```python
from build123d import *

# Parameters (mm, degrees)
SKETCH_1_W          = 20
SKETCH_1_H          = 30
SKETCH_1_W_2        = 18
SKETCH_1_H_2        = 28
EXTRUDE_1_DEPTH     = 105
CUT_EXTRUDE_1_REACH = 111.659
SKETCH_2_R          = 1.5
CUT_EXTRUDE_3_REACH = 109.935
SKETCH_5_R          = 11


with BuildPart() as part:
    # 草图1 → 拉伸-薄壁1 (new body)
    with BuildSketch(Plane.XY):
        Rectangle(SKETCH_1_W, SKETCH_1_H)
        Rectangle(SKETCH_1_W_2, SKETCH_1_H_2, mode=Mode.SUBTRACT)
    extrude(amount=EXTRUDE_1_DEPTH)

    # 切除-拉伸1: up to this face of the body (flat: up to its plane)
    cut_extrude_1_end = Plane(part.part.faces().sort_by_distance((0, -15, 52.5))[0])
    # 草图2 → 切除-拉伸1 (cut, up to the picked face)
    with BuildSketch(Plane(origin=(0, 15, 0), x_dir=(1, 0, 0), z_dir=(0, 1, 0)), mode=Mode.PRIVATE) as cut_extrude_1_sk1:
        with Locations(Location((5, -10, 0), (0, 0, 270))):
            Circle(SKETCH_2_R)
    cut_extrude_1_tool1 = split(extrude(cut_extrude_1_sk1.sketch, amount=-CUT_EXTRUDE_1_REACH, mode=Mode.PRIVATE), bisect_by=cut_extrude_1_end, keep=Keep.BOTH, mode=Mode.PRIVATE)
    # 草图2 → 切除-拉伸1 (cut, up to the picked face)
    with BuildSketch(Plane(origin=(0, 15, 0), x_dir=(1, 0, 0), z_dir=(0, 1, 0)), mode=Mode.PRIVATE) as cut_extrude_1_sk2:
        with Locations(Location((-5, -10, 0), (0, 0, 270))):
            Circle(SKETCH_2_R)
    cut_extrude_1_tool2 = split(extrude(cut_extrude_1_sk2.sketch, amount=-CUT_EXTRUDE_1_REACH, mode=Mode.PRIVATE), bisect_by=cut_extrude_1_end, keep=Keep.BOTH, mode=Mode.PRIVATE)
    # 草图2 → 切除-拉伸1 (cut, up to the picked face)
    with BuildSketch(Plane(origin=(0, 15, 0), x_dir=(1, 0, 0), z_dir=(0, 1, 0)), mode=Mode.PRIVATE) as cut_extrude_1_sk3:
        with Locations(Location((5, -95, 0), (0, 0, 270))):
            Circle(SKETCH_2_R)
    cut_extrude_1_tool3 = split(extrude(cut_extrude_1_sk3.sketch, amount=-CUT_EXTRUDE_1_REACH, mode=Mode.PRIVATE), bisect_by=cut_extrude_1_end, keep=Keep.BOTH, mode=Mode.PRIVATE)
    # 草图2 → 切除-拉伸1 (cut, up to the picked face)
    with BuildSketch(Plane(origin=(0, 15, 0), x_dir=(1, 0, 0), z_dir=(0, 1, 0)), mode=Mode.PRIVATE) as cut_extrude_1_sk4:
        with Locations(Location((-5, -95, 0), (0, 0, 270))):
            Circle(SKETCH_2_R)
    cut_extrude_1_tool4 = split(extrude(cut_extrude_1_sk4.sketch, amount=-CUT_EXTRUDE_1_REACH, mode=Mode.PRIVATE), bisect_by=cut_extrude_1_end, keep=Keep.BOTH, mode=Mode.PRIVATE)
    add(cut_extrude_1_tool1.solids().sort_by(Axis((5, 15, 10), (0, -1, 0)))[0], mode=Mode.SUBTRACT)
    add(cut_extrude_1_tool2.solids().sort_by(Axis((-5, 15, 10), (0, -1, 0)))[0], mode=Mode.SUBTRACT)
    add(cut_extrude_1_tool3.solids().sort_by(Axis((5, 15, 95), (0, -1, 0)))[0], mode=Mode.SUBTRACT)
    add(cut_extrude_1_tool4.solids().sort_by(Axis((-5, 15, 95), (0, -1, 0)))[0], mode=Mode.SUBTRACT)

    # 切除-拉伸3: up to this face of the body (flat: up to its plane)
    cut_extrude_3_end = Plane(part.part.faces().sort_by_distance((-10, 0, 52.5))[0])
    # 草图5 → 切除-拉伸3 (cut, up to the picked face)
    with BuildSketch(Plane(origin=(10, 0, 0), x_dir=(0, 0, -1), z_dir=(1, 0, 0)), mode=Mode.PRIVATE) as cut_extrude_3_sk1:
        with Locations((-20, 0)):
            Circle(SKETCH_5_R)
    cut_extrude_3_tool1 = split(extrude(cut_extrude_3_sk1.sketch, amount=-CUT_EXTRUDE_3_REACH, mode=Mode.PRIVATE), bisect_by=cut_extrude_3_end, keep=Keep.BOTH, mode=Mode.PRIVATE)
    # 草图5 → 切除-拉伸3 (cut, up to the picked face)
    with BuildSketch(Plane(origin=(10, 0, 0), x_dir=(0, 0, -1), z_dir=(1, 0, 0)), mode=Mode.PRIVATE) as cut_extrude_3_sk2:
        with Locations((-52.5, 0)):
            Circle(SKETCH_5_R)
    cut_extrude_3_tool2 = split(extrude(cut_extrude_3_sk2.sketch, amount=-CUT_EXTRUDE_3_REACH, mode=Mode.PRIVATE), bisect_by=cut_extrude_3_end, keep=Keep.BOTH, mode=Mode.PRIVATE)
    # 草图5 → 切除-拉伸3 (cut, up to the picked face)
    with BuildSketch(Plane(origin=(10, 0, 0), x_dir=(0, 0, -1), z_dir=(1, 0, 0)), mode=Mode.PRIVATE) as cut_extrude_3_sk3:
        with Locations((-85, 0)):
            Circle(SKETCH_5_R)
    cut_extrude_3_tool3 = split(extrude(cut_extrude_3_sk3.sketch, amount=-CUT_EXTRUDE_3_REACH, mode=Mode.PRIVATE), bisect_by=cut_extrude_3_end, keep=Keep.BOTH, mode=Mode.PRIVATE)
    add(cut_extrude_3_tool1.solids().sort_by(Axis((10, 0, 20), (-1, 0, 0)))[0], mode=Mode.SUBTRACT)
    add(cut_extrude_3_tool2.solids().sort_by(Axis((10, 0, 52.5), (-1, 0, 0)))[0], mode=Mode.SUBTRACT)
    add(cut_extrude_3_tool3.solids().sort_by(Axis((10, 0, 85), (-1, 0, 0)))[0], mode=Mode.SUBTRACT)


solid = part.part
```
The model under review builds one solid part; all positions refer to its coordinate system, in mm. A direction names the side the tool comes from. Round coordinates to 2 decimals unless told otherwise and drop trailing zeros. Loops run counter-clockwise (first coordinate to the right, second up) from the corner with the lowest first, then second, coordinate; pieces in that order, holes last.
Item 1: Take a section at C-C (z = 20). Write out the cut boundary in (x, y), then the cut area to 3 significant figures.
Determined:
outline: (-10, -15) - (10, -15) - (10, -11) - (9, -11) - (9, -14) - (-9, -14) - (-9, -11) - (-10, -11) - close; (-10, 11) - (-9, 11) - (-9, 14) - (9, 14) - (9, 11) - (10, 11) - (10, 15) - (-10, 15) - close
area: 52.0 mm2
Item 2: Mouldability with a two-part tool opening along Z and no side actions: class faces 1 (the face through (5.07, 14.51, 8.5)), 2 (the face through (-9.7, 0.1, 105)), 3 (the face through (0, 15, 52)) as released by +Z, released by -Z, zero draft, split by the parting line, or undercut.
Determined:
face 1: undercut
face 2: released by +Z
face 3: zero draft
Item 3: For faces 4 (the face through (-9, 2.9, 63.4)), 5 (the face through (0, -15, 52)), list the 3-axis set-ups (+Z, -Z, +X, -X, +Y, -Y) from which the entire face can be reached by the end or side of a thin tool; tool diameter is ignored.
Determined:
face 4: +Z, -Z
face 5: +Z, -Z, +X, -X, -Y
Item 4: Clearance check with flat-ended pins moving along their axes: pin 1 Ø17.5 at (y, z) = (0, 52.5) entering from +X; pin 2 Ø3.5 at (x, z) = (5, 95) entering from +Y. State where each tip first meets the part, or that it passes through.
Determined:
pin 1: passes through
pin 2: stops at y = 15
Item 5: Take a section at B-B (y = 0). Give the number of separate pieces and of enclosed holes in the cut face, then the cut area to 3 significant figures.
Determined:
separate pieces: 8
enclosed holes: 0
area: 78.0 mm2
Item 6: Take a section at D-D (x = 1). Write out the cut boundary in (y, z), then the cut area to 3 significant figures.
Determined:
outline: (-15, 0) - (-14, 0) - (-14, 105) - (-15, 105) - close; (14, 0) - (15, 0) - (15, 105) - (14, 105) - close
area: 210 mm2
Item 7: Take a section at A-A (x = -5). Write out the cut boundary in (y, z).
Determined:
outline: (-15, 0) - (-14, 0) - (-14, 8.5) - (-15, 8.5) - close; (-15, 11.5) - (-14, 11.5) - (-14, 93.5) - (-15, 93.5) - close; (-15, 96.5) - (-14, 96.5) - (-14, 105) - (-15, 105) - close; (14, 0) - (15, 0) - (15, 8.5) - (14, 8.5) - close; (14, 11.5) - (15, 11.5) - (15, 93.5) - (14, 93.5) - close; (14, 96.5) - (15, 96.5) - (15, 105) - (14, 105) - close
Item 8: For line 1 (X direction, y = -0.25, z = 71.5); line 2 (X direction, y = 14.45, z = 10); line 3 (Y direction, x = 5, z = 56), list the stretches that pass through material, from the lowest coordinate up.
Determined:
line 1: x = -10 to -9, 9 to 10
line 2: x = -10 to -6.5, -3.5 to 3.5, 6.5 to 10
line 3: y = -15 to -14, 14 to 15
